from build123d import *

# Parameters (mm, degrees)
TROU_TARAUD_M31_D     = 2.5
TROU_TARAUD_M31_DEPTH = 8
TROU_TARAUD_M31_TIP   = 0.751075774
ESQUISSE7_W           = 5
ESQUISSE7_H           = 0.5
CHANFREIN1_SIZE       = 0.2
TROU_TARAUD_M32_D     = 2.5
TROU_TARAUD_M32_DEPTH = 8
TROU_TARAUD_M32_TIP   = 0.751075774


with BuildPart() as part:
    # Esquisse2 → Révolution1 (revolve)
    with BuildSketch(Plane.XY, mode=Mode.PRIVATE) as r_volution1_sk:
        Polygon((17, 0), (17, 2.5), (-0.5, 2.5), (-0.5, 3), (-17, 3), (-17, 0), align=None)
    revolve(r_volution1_sk.sketch.rotate(Axis((-17, 0, 0), (1, 0, 0)), 90), axis=Axis((-17, 0, 0), (1, 0, 0)))

    # Trou taraudé M31
    with Locations(Plane(origin=(17, 0, 0), x_dir=(0, 0, -1), z_dir=(1, 0, 0))):
        with Locations((0, 0)):
            Hole(TROU_TARAUD_M31_D / 2, depth=TROU_TARAUD_M31_DEPTH)
            with Locations((0, 0, -(TROU_TARAUD_M31_DEPTH + TROU_TARAUD_M31_TIP / 2))):  # 118° drill point
                Cone(0, TROU_TARAUD_M31_D / 2, TROU_TARAUD_M31_TIP, mode=Mode.SUBTRACT)

    # Esquisse7 → Enlèvement de matière-Révolution1 (revolve, cut)
    with BuildSketch(Plane.XY, mode=Mode.PRIVATE) as enl_vement_de_mati_re_r_volution1_sk:
        with Locations((-14.5, 2.75)):
            Rectangle(ESQUISSE7_W, ESQUISSE7_H)
    revolve(enl_vement_de_mati_re_r_volution1_sk.sketch.rotate(Axis((-17, 0, 0), (1, 0, 0)), 90), axis=Axis((-17, 0, 0), (1, 0, 0)), mode=Mode.SUBTRACT)

    # Chanfrein1
    chanfrein1_edges = [part.edges().sort_by_distance(p)[0] for p in [
        (-17, 0, -2.5),
        (17, 0, -2.5),
    ]]
    chamfer(chanfrein1_edges, length=CHANFREIN1_SIZE)

    # Trou taraudé M32
    with Locations(Plane.ZY.offset(17)):
        with Locations((0, 0)):
            Hole(TROU_TARAUD_M32_D / 2, depth=TROU_TARAUD_M32_DEPTH)
            with Locations((0, 0, -(TROU_TARAUD_M32_DEPTH + TROU_TARAUD_M32_TIP / 2))):  # 118° drill point
                Cone(0, TROU_TARAUD_M32_D / 2, TROU_TARAUD_M32_TIP, mode=Mode.SUBTRACT)


solid = part.part
Work out the finished part from the listing and answer in its coordinate system (mm). A direction names the side the tool comes from. Give positions to 0.01 mm unless a question says otherwise; leave off trailing zeros. Order: outer loops, then holes, each group sorted by start corner. A loop starts at its lowest first (then second) coordinate and runs counter-clockwise, first axis right, second up. Notation, with made-up numbers: (34, -12) -> (67, -12) arc R26 ccw to (67, 22) -> close; hole circle Ø9 at (-32, 11.25). An arc over 180 degrees is marked (long way). One line per item, written item: value.
Item 1: Straight lines are drawn through the part: probe 1 along Y at (x, z) = (-11.5, 0); probe 2 along Y at (x, z) = (-13.25, 0); probe 3 along Z at (x, y) = (-8.5, 0.1). For each, find the intervals that lie inside material, in ascending order.
Answer sheet:
probe 1: -3 to -1.25, 1.25 to 3
probe 2: -2.5 to -1.25, 1.25 to 2.5
probe 3: -3 to -0.41, 0.41 to 3
Item 2: Find section A-A, the plane x = -4. Give the vertices of the cut face in (y, z).
Answer sheet:
outline: circle Ø6 at (0, 0)
Item 3: Find section B-B, the plane x = 2.5. Give the vertices of the cut face in (y, z), plus the area to 3 significant figures.
Answer sheet:
outline: circle Ø5 at (0, 0)
area: 19.6 mm²
Item 4: Flat-ended cylindrical pins translate along their axes: P1, Ø1.5, axis at y = 0, z = 0, coming from the -X side; P2, Ø1, axis at x = -11, y = -1, coming from the -Z side. Find the tip coordinate at first contact, or state that the pin passes through.
Answer sheet:
P1: x = -8.7
P2: z = -2.96
Item 5: A tool of negligible diameter and unlimited length cuts with its end or side. For faces 5 (the cylindrical face through (-12.94, -1.22, 0.27)), 6 (the flat face through (-17, 1, 1)), 7 (the cylindrical face through (8, -0.1, -2.5)), from which of +Z, -Z, +X, -X, +Y, -Y can it reach the whole face along a straight path? Write none if from no direction.
Answer sheet:
face 5: -X
face 6: +Z, -Z, -X, +Y, -Y
face 7: +X
Item 6: Determine the mould class of faces 1 (the flat face through (17, 1, -1)), 2 (the cylindrical face through (12.94, -1.22, -0.27)), 3 (the conical face through (-8.38, -0.21, -0.05)), 4 (the cylindrical face through (-6.33, -0.9, 2.86)) for opening direction Z: released by +Z, released by -Z, zero draft, split by the parting line, or undercut.
Answer sheet:
face 1: zero draft
face 2: undercut
face 3: undercut
face 4: split by the parting line
